```python
from build123d import *

# Parameters (mm, degrees)
SKETCH1_W           = 2
SKETCH1_H           = 40
SKETCH1_W_2         = 38
SKETCH1_H_2         = 2
SKETCH1_H_3         = 4.5
WALLS_DEPTH         = 20
SKETCH1_3_W         = 4.5
SKETCH1_3_H         = 40
SKETCH1_3_H_2       = 2
REST_ON_THIS_DEPTH  = 2
SKETCH2_W           = 10
SKETCH2_H           = 10
SKETCH2_R           = 2.5
BOSS_EXTRUDE3_DEPTH = 2


with BuildPart() as part:
    # Sketch1 → Walls (new body)
    with BuildSketch(Plane(origin=(0, 0, 0), x_dir=(1, 0, 0), z_dir=(0, 1, 0))):
        with Locations((-19.503168436, 5.037980983)):
            Rectangle(SKETCH1_W, SKETCH1_H)
        with Locations((-13.003168436, 5.037980983)):
            Rectangle(SKETCH1_W, SKETCH1_H)
        Polygon((-12.003168436, -14.962019017), (-14.003168436, -14.962019017), (-14.003168436, -16.962019017), (19.496831564, -16.962019017), (25.996831564, -16.962019017), (25.996831564, -14.962019017), align=None)
        with Locations((0.496831564, -22.462019017)):
            Rectangle(SKETCH1_W_2, SKETCH1_H_2)
        with Locations((-19.503168436, -22.462019017)):
            Rectangle(SKETCH1_W, SKETCH1_H_2)
        with Locations((-19.503168436, -19.212019017)):
            Rectangle(SKETCH1_W, SKETCH1_H_3)
        with Locations((-19.503168436, -15.962019017)):
            Rectangle(SKETCH1_W, SKETCH1_H_2)
    extrude(amount=-WALLS_DEPTH)

    # Sketch1_3 → Rest on this (add)
    with BuildSketch(Plane(origin=(0, 0, 0), x_dir=(1, 0, 0), z_dir=(0, 1, 0))):
        with Locations((-16.253168436, 5.037980983)):
            Rectangle(SKETCH1_3_W, SKETCH1_3_H)
        with Locations((-16.253168436, -15.962019017)):
            Rectangle(SKETCH1_3_W, SKETCH1_3_H_2)
        Polygon((-14.003168436, -16.962019017), (-18.503168436, -16.962019017), (-18.503168436, -21.462019017), (19.496831564, -21.462019017), (19.496831564, -16.962019017), align=None)
    extrude(amount=-REST_ON_THIS_DEPTH)

    # Sketch2 → Boss-Extrude3 (add)
    # profile 1 of 3: a face of its own
    with BuildSketch(Plane(origin=(0, 0, 0), x_dir=(1, 0, 0), z_dir=(0, 1, 0))):
        Polygon((7.996831564, -14.962019017), (-12.003168436, 5.037980983), (-12.003168436, -14.962019017), align=None)
    # profile 2 of 3: a face of its own
    with BuildSketch(Plane(origin=(0, 0, 0), x_dir=(1, 0, 0), z_dir=(0, 1, 0))):
        with Locations((14.496831564, -28.462019017)):
            Rectangle(SKETCH2_W, SKETCH2_H)
        with Locations(Location((14.496831564, -28.462019017, 0), (0, 0, 270))):
            Circle(SKETCH2_R, mode=Mode.SUBTRACT)
    # profile 3 of 3: a face of its own
    with BuildSketch(Plane(origin=(0, 0, 0), x_dir=(1, 0, 0), z_dir=(0, 1, 0))):
        with Locations((-25.503168436, 20.037980983)):
            Rectangle(SKETCH2_W, SKETCH2_H)
        with Locations(Location((-25.503168436, 20.037980983, 0), (0, 0, 270))):
            Circle(SKETCH2_R, mode=Mode.SUBTRACT)
    extrude(amount=-BOSS_EXTRUDE3_DEPTH)


solid = part.part
```
Work out the finished part from the listing and answer in its coordinate system (mm). A direction names the side the tool comes from. Give positions to 0.01 mm unless a question says otherwise; leave off trailing zeros. Loops run counter-clockwise (first coordinate to the right, second up) from the corner with the lowest first, then second, coordinate; pieces in that order, holes last. Notation, with made-up numbers: (23.5, 26.5) -> (79.5, 26.5) arc R23 cw to (79.5, 47.5) -> close; hole circle Ø1 at (19, 3.5). An arc over 180 degrees is marked (long way). Use CSV: the item, a comma, the result in double quotes.
1. Straight lines are drawn through the part: line 1 (X direction, y = -5.5, z = 10); line 2 (X direction, y = -10, z = 15); line 3 (Z direction, x = 8.5, y = -9.25). For each, find the intervals that lie inside material, in ascending order.
Found:
line 1,"-20.5 to -18.5, -14 to -12"
line 2,"-20.5 to -18.5, -14 to 26"
line 3,"14.96 to 16.96, 21.46 to 23.46"
2. The part is cut by section D-D (x = 5.5). Write down the section's boundary in (y, z), then the cut area to 3 significant figures.
Found:
outline,"(-20, 14.96) -> (-2, 14.96) -> (-2, 12.47) -> (0, 12.47) -> (0, 23.46) -> (-20, 23.46) -> (-20, 21.46) -> (-2, 21.46) -> (-2, 16.96) -> (-20, 16.96) -> close"
area,"94.0 mm^2"
3. A tool of negligible diameter and unlimited length cuts with its end or side. For faces 5 (the flat face through (12, -2, 27)), 6 (the flat face through (-26, -1, -15.038)), 7 (the flat face through (-14.003, -11, -4)), 8 (the flat face through (-12.003, -10, -5)), 9 (the flat face through (19.497, -7, 23)), from which of +Z, -Z, +X, -X, +Y, -Y can it reach the whole face along a straight path? Write none if from no direction.
Found:
face 5,"+Z, +X, -X, -Y"
face 6,"+Z, -X, +Y, -Y"
face 7,"-Z, -Y"
face 8,"-Z, +X, -Y"
face 9,"+Z, +X, +Y, -Y"
4. The part is cut by section C-C (z = -8). Write down the section's boundary in (x, y).
Found:
outline,"(-20.5, -20) -> (-18.5, -20) -> (-18.5, -2) -> (-14, -2) -> (-14, -20) -> (-12, -20) -> (-12, 0) -> (-20.5, 0) -> close"
5. The part is cut by section A-A (y = -18). Write down the section's boundary in (x, z).
Found:
outline,"(-20.5, -25.04) -> (-18.5, -25.04) -> (-18.5, 21.46) -> (19.5, 21.46) -> (19.5, 23.46) -> (-20.5, 23.46) -> close; (-14, -25.04) -> (-12, -25.04) -> (-12, 14.96) -> (26, 14.96) -> (26, 16.96) -> (-14, 16.96) -> close"
6. The part is cut by section B-B (z = -20.5). Write down the section's boundary in (x, y), then the cut area to 3 significant figures.
Found:
outline,"(-30.5, -2) -> (-27.96, -2) -> (-27.96, 0) -> (-30.5, 0) -> close; (-23.05, -2) -> (-20.5, -2) -> (-20.5, -20) -> (-18.5, -20) -> (-18.5, -2) -> (-14, -2) -> (-14, -20) -> (-12, -20) -> (-12, 0) -> (-23.05, 0) -> close"
area,"99.2 mm^2"
7. The mould has two halves that part along X. Classify faces 1 (the flat face through (14, -1, 33.462)), 2 (the flat face through (25.997, -10, 16)), 3 (the cylindrical face through (16.19, -0.99, 26.62)), 4 (the flat face through (-15, -2, 8)): +X half, -X half, draft (parallel to the pull), parting line (faces both ways), or undercut.
Found:
face 1,"draft"
face 2,"+X half"
face 3,"undercut"
face 4,"undercut"
8. Flat-ended cylindrical pins translate along their axes: pin 1 Ø6 at (x, y) = (-25, -7) entering from +Z; pin 2 Ø9 at (y, z) = (-7, -12) entering from -X; pin 3 Ø6 at (x, z) = (-25.5, -20.04) entering from -Y; pin 4 Ø22 at (x, z) = (-3.5, 1) entering from -Y. Find the tip coordinate at first contact, or state that the pin passes through.
Found:
pin 1,"through"
pin 2,"x = -20.5"
pin 3,"y = -2"
pin 4,"y = -20"
